Could you check a few things on this model? Use its own coordinates, in mm. Face numbers are marked on the shaded views. A direction names the side the tool comes from. Give positions to 0.01 mm unless a question says otherwise; leave off trailing zeros. Loops run counter-clockwise (first coordinate to the right, second up) from the corner with the lowest first, then second, coordinate; pieces in that order, holes last.
1. Imagine slicing it at D-D (x = -1.75). List the corners of the cut face in (y, z) for me, plus the area to 3 significant figures.
2. I need wall thicknesses on line 1 along X through (y, z) = (-2.5, 3.25); line 2 along Z through (x, y) = (-0.75, -1.75); line 3 along Z through (x, y) = (3.75, -2.25). Which ranges of each line are inside material? Lowest first, please.
3. Thinking about a two-plate mould opening in Y: for the marked faces 1, 2 and 3, which applies, +Y half, -Y half, draft (parallel to the pull), parting line (faces both ways), or undercut?
4. For P1, Ø2, axis at x = 3.5, y = 2.5, coming from the +Z side; P2, Ø1, axis at x = -1.5, y = 2, coming from the +Z side; P3, Ø6, axis at x = -1, y = -3.5, coming from the +Z side, each with a flat end and sliding along its axis, tell me the tip position at first contact or that it passes through.
5. Imagine slicing it at A-A (x = -4.5). List the corners of the cut face in (y, z) for me, plus the area to 3 significant figures.
6. For the marked faces 4, 5 and 6, which set-ups out of +Z, -Z, +X, -X, +Y, -Y let a thin tool reach every point of the face, with its end or its side?
7. Imagine slicing it at B-B (z = 1.25). List the corners of the cut face in (x, y) for me, plus the area to 3 significant figures.
```python
from build123d import *

# Parameters (mm, degrees)
CUT_EXTRUDE1_DEPTH      = 14.076696831
CUT_EXTRUDE2_DEPTH      = 10.105317074
CUT_EXTRUDE2_DEPTH_BACK = 10.105317074
SKETCH4_R               = 0.5


with BuildPart() as part:
    # Sketch1 → Revolve1 (revolve)
    with BuildSketch(Plane(origin=(0, 0, 0), x_dir=(1, 0, 0), z_dir=(0, 1, 0))):
        Polygon((-3.5, -5), (-3.5, -4), (3.5, -4), (3.5, -5), (5.5, -5), (5.5, 0), (-5.5, 0), (-5.5, -5), align=None)
    revolve(axis=Axis((-5.5, 0, 0), (1, 0, 0)))

    # Sketch3 → Cut-Extrude1 (cut, through all)
    with BuildSketch(Plane(origin=(5.5, 0, 0), x_dir=(0, 0, -1), z_dir=(1, 0, 0))):
        with BuildLine():
            ThreePointArc((0.110278314, 2.697746966), (-0.12087287, 2.635504953), (-0.275087283, 2.452412483))
            Line((-0.275087283, 2.452412483), (-0.566923139, 1.754593444))
            ThreePointArc((-0.566923139, 1.754593444), (-0.675530556, 1.646723678), (-0.82860304, 1.647245277))
            Line((-0.82860304, 1.647245277), (-1.526422079, 1.939081132))
            ThreePointArc((-1.526422079, 1.939081132), (-1.764789364, 1.961125979), (-1.973058824, 1.843105769))
            ThreePointArc((-1.973058824, 1.843105769), (-2.490939467, 1.041739204), (-2.697746966, 0.110278314))
            ThreePointArc((-2.697746966, 0.110278314), (-2.635504953, -0.12087287), (-2.452412483, -0.275087283))
            Line((-2.452412483, -0.275087283), (-1.754593444, -0.566923139))
            ThreePointArc((-1.754593444, -0.566923139), (-1.646723678, -0.675530556), (-1.647245277, -0.82860304))
            Line((-1.647245277, -0.82860304), (-1.939081132, -1.526422079))
            ThreePointArc((-1.939081132, -1.526422079), (-1.961125979, -1.764789364), (-1.843105769, -1.973058824))
            ThreePointArc((-1.843105769, -1.973058824), (-1.041739204, -2.490939467), (-0.110278314, -2.697746966))
            ThreePointArc((-0.110278314, -2.697746966), (0.12087287, -2.635504953), (0.275087283, -2.452412483))
            Line((0.275087283, -2.452412483), (0.566923139, -1.754593444))
            ThreePointArc((0.566923139, -1.754593444), (0.675530556, -1.646723678), (0.82860304, -1.647245277))
            Line((0.82860304, -1.647245277), (1.526422079, -1.939081132))
            ThreePointArc((1.526422079, -1.939081132), (1.764789364, -1.961125979), (1.973058824, -1.843105769))
            ThreePointArc((1.973058824, -1.843105769), (2.490939467, -1.041739204), (2.697746966, -0.110278314))
            ThreePointArc((2.697746966, -0.110278314), (2.635504953, 0.12087287), (2.452412483, 0.275087283))
            Line((2.452412483, 0.275087283), (1.754593444, 0.566923139))
            ThreePointArc((1.754593444, 0.566923139), (1.646723678, 0.675530556), (1.647245277, 0.82860304))
            Line((1.647245277, 0.82860304), (1.939081132, 1.526422079))
            ThreePointArc((1.939081132, 1.526422079), (1.961125979, 1.764789364), (1.843105769, 1.973058824))
            ThreePointArc((1.843105769, 1.973058824), (1.041739204, 2.490939467), (0.110278314, 2.697746966))
        make_face()
    extrude(amount=-CUT_EXTRUDE1_DEPTH, mode=Mode.SUBTRACT)

    # Sketch4 → Cut-Extrude2 (cut, two sides: drawn at the far end of the back side and taken through both)
    with BuildSketch(Plane(origin=(0, 0.077165867, 0.184514035), x_dir=(-1, 0, 0), z_dir=(0, -0.38582933492302907, -0.9225701731103457)).offset(-CUT_EXTRUDE2_DEPTH_BACK)):
        with Locations(Location((0, 0, 0), (0, 0, 90))):
            Circle(SKETCH4_R)
    extrude(amount=CUT_EXTRUDE2_DEPTH + CUT_EXTRUDE2_DEPTH_BACK, mode=Mode.SUBTRACT)


solid = part.part
```
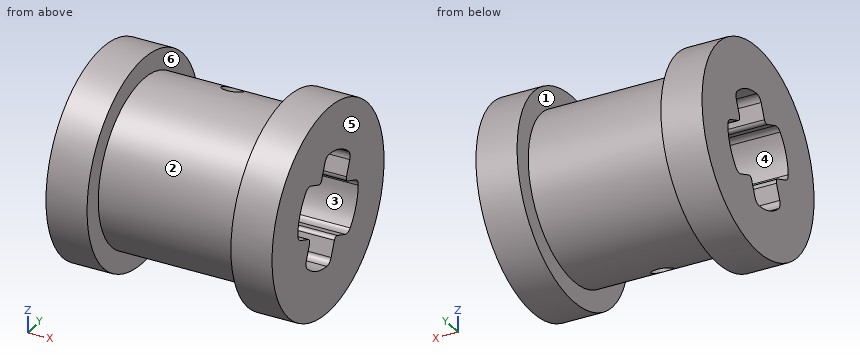
Derived:
1. outline: circle Ø8 at (0, 0); hole (-2.7, 0.11) arc R0.4 ccw to (-2.45, -0.28) - (-1.75, -0.57) arc R0.2 cw to (-1.65, -0.83) - (-1.94, -1.53) arc R0.4 ccw to (-1.84, -1.97) arc R2.7 ccw to (-0.11, -2.7) arc R0.4 ccw to (0.28, -2.45) - (0.57, -1.75) arc R0.2 cw to (0.83, -1.65) - (1.53, -1.94) arc R0.4 ccw to (1.97, -1.84) arc R2.7 ccw to (2.7, -0.11) arc R0.4 ccw to (2.45, 0.28) - (1.75, 0.57) arc R0.2 cw to (1.65, 0.83) - (1.94, 1.53) arc R0.4 ccw to (1.84, 1.97) arc R2.7 ccw to (0.11, 2.7) arc R0.4 ccw to (-0.28, 2.45) - (-0.57, 1.75) arc R0.2 cw to (-0.83, 1.65) - (-1.53, 1.94) arc R0.4 ccw to (-1.97, 1.84) arc R2.7 ccw to start
1. area: 31.1 mm2
2. line 1: x = -5.5 to -3.5, 3.5 to 5.5
2. line 2: z = -3.6 to -2.06, -1.07 to -0.57, 1.96 to 3.6
2. line 3: z = -4.47 to -0.36, 1.49 to 4.47
3. face 1: draft
3. face 2: parting line
3. face 3: undercut
4. P1: stops at z = 4.77
4. P2: stops at z = 3.71
4. P3: stops at z = 4.65
5. outline: circle Ø10 at (0, 0); hole (-2.7, 0.11) arc R0.4 ccw to (-2.45, -0.28) - (-1.75, -0.57) arc R0.2 cw to (-1.65, -0.83) - (-1.94, -1.53) arc R0.4 ccw to (-1.84, -1.97) arc R2.7 ccw to (-0.11, -2.7) arc R0.4 ccw to (0.28, -2.45) - (0.57, -1.75) arc R0.2 cw to (0.83, -1.65) - (1.53, -1.94) arc R0.4 ccw to (1.97, -1.84) arc R2.7 ccw to (2.7, -0.11) arc R0.4 ccw to (2.45, 0.28) - (1.75, 0.57) arc R0.2 cw to (1.65, 0.83) - (1.94, 1.53) arc R0.4 ccw to (1.84, 1.97) arc R2.7 ccw to (0.11, 2.7) arc R0.4 ccw to (-0.28, 2.45) - (-0.57, 1.75) arc R0.2 cw to (-0.83, 1.65) - (-1.53, 1.94) arc R0.4 ccw to (-1.97, 1.84) arc R2.7 ccw to start
5. area: 59.3 mm2
6. face 4: +X, -X
6. face 5: +Z, -Z, +X, +Y, -Y
6. face 6: none
7. outline: (-5.5, -4.84) - (-3.5, -4.84) - (-3.5, -3.8) - (3.5, -3.8) - (3.5, -4.84) - (5.5, -4.84) - (5.5, -2.39) - (-5.5, -2.39) - close; (-5.5, 1.82) - (5.5, 1.82) - (5.5, 4.84) - (3.5, 4.84) - (3.5, 3.8) - (-3.5, 3.8) - (-3.5, 4.84) - (-5.5, 4.84) - close
7. area: 45.5 mm2
